The listing builds one solid part. Answer for the finished solid, in the listing's coordinates (mm). Face numbers are marked on the shaded views. A direction names the side the tool comes from. Give positions to 0.01 mm unless a question says otherwise; leave off trailing zeros. Write each loop counter-clockwise with the first axis right and the second up, starting at its lowest first coordinate (ties: lowest second). Pieces come first, ordered by that corner, then holes. Notation, with made-up numbers: (72.5, 50) - (118.5, 50) arc R16 ccw to (118.5, 77) - close; hole circle Ø1 at (71.25, -9). An arc over 180 degrees is marked (long way). Return JSON: item names as keys, results as strings.
from build123d import *

# Parameters (mm, degrees)
SKETCH1_R           = 55.88
BOSS_EXTRUDE1_DEPTH = 23.495
SKETCH2_R           = 66.675
BOSS_EXTRUDE2_DEPTH = 13.97
FILLET1_R           = 7.62
SKETCH3_R           = 2.8575
CUT_EXTRUDE1_DEPTH  = 38.465
CIRPATTERN1_COUNT   = 8
SKETCH4_R           = 38.735
CUT_EXTRUDE2_DEPTH  = 10.795
SKETCH5_R           = 34.4043
CUT_EXTRUDE3_DEPTH  = 40.894


with BuildPart() as part:
    # Sketch1 → Boss-Extrude1 (new body)
    with BuildSketch(Plane(origin=(0, 0, 0), x_dir=(1, 0, 0), z_dir=(0, 1, 0))):
        Circle(SKETCH1_R)
    extrude(amount=BOSS_EXTRUDE1_DEPTH)

    # Sketch2 → Boss-Extrude2 (add)
    with BuildSketch(Plane(origin=(0, 23.495, 0), x_dir=(1, 0, 0), z_dir=(0, 1, 0))):
        Circle(SKETCH2_R)
    extrude(amount=BOSS_EXTRUDE2_DEPTH)

    # Fillet1
    fillet1_edges = [part.edges().sort_by_distance(p)[0] for p in [
        (-55.88, 23.495, 0),
    ]]
    fillet(fillet1_edges, radius=FILLET1_R)

    # Sketch3 → Cut-Extrude1 (cut, through all)
    with BuildSketch(Plane(origin=(0, 37.465, 0), x_dir=(1, 0, 0), z_dir=(0, 1, 0))):
        with Locations((0, 61.2775)):
            Circle(SKETCH3_R)
    cut_extrude1 = extrude(amount=-CUT_EXTRUDE1_DEPTH, mode=Mode.SUBTRACT)

    # CirPattern1: Cut-Extrude1 ×8 about axis
    cirpattern1_axis = Axis((0, 0, 0), (0, 1, 0))
    for i in range(1, CIRPATTERN1_COUNT):
        add(cut_extrude1.rotate(cirpattern1_axis, i * 360 / CIRPATTERN1_COUNT), mode=Mode.SUBTRACT)

    # Sketch4 → Cut-Extrude2 (cut)
    with BuildSketch(Plane(origin=(0, 37.465, 0), x_dir=(1, 0, 0), z_dir=(0, 1, 0))):
        Circle(SKETCH4_R)
    extrude(amount=-CUT_EXTRUDE2_DEPTH, mode=Mode.SUBTRACT)

    # Sketch5 → Cut-Extrude3 (cut)
    with BuildSketch(Plane(origin=(0, 26.67, 0), x_dir=(1, 0, 0), z_dir=(0, 1, 0))):
        Circle(SKETCH5_R)
    extrude(amount=-CUT_EXTRUDE3_DEPTH, mode=Mode.SUBTRACT)


solid = part.part
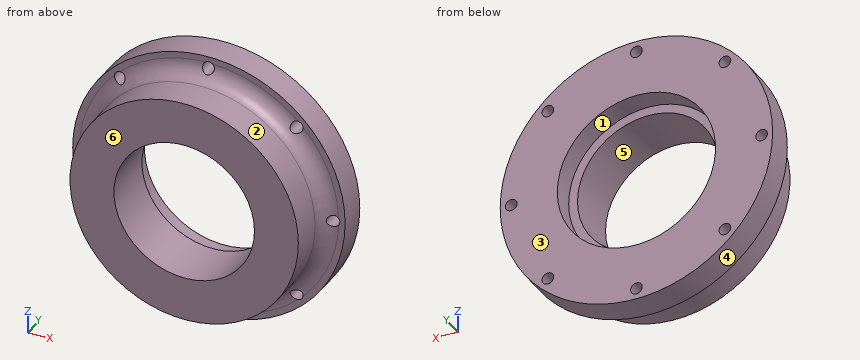
Item 1: Consider L1, parallel to Z at x = 0, y = 30.5 (3 decimals); L2, parallel to X at y = 26, z = 0 (3 decimals). Determine where each line is inside the solid, lowest interval first.
Answer below:
{"L1": "z = -66.675 to -64.135, -58.42 to -38.735, 38.735 to 58.42, 64.135 to 66.675", "L2": "x = -66.675 to -64.135, -58.42 to -34.404, 34.404 to 58.42, 64.135 to 66.675"}
Item 2: The mould has two halves that part along X. Classify the marked faces 4, 5 and 6: +X half, -X half, draft (parallel to the pull), parting line (faces both ways), or undercut.
Answer below:
{"face 4": "parting line", "face 5": "undercut", "face 6": "draft"}
Item 3: A cutting plane is placed at B-B on z = 0. Determine the outline of the cut face in (x, y) (3 decimals), then the cut area to 3 significant figures.
Answer below:
{"outline": "(-66.675, 23.495) - (-64.135, 23.495) - (-64.135, 37.465) - (-66.675, 37.465) - close; (-58.42, 21.555) arc R7.62 cw to (-55.88, 15.875) - (-55.88, 0) - (-34.404, 0) - (-34.404, 26.67) - (-38.735, 26.67) - (-38.735, 37.465) - (-58.42, 37.465) - close; (34.404, 0) - (55.88, 0) - (55.88, 15.875) arc R7.62 cw to (58.42, 21.555) - (58.42, 37.465) - (38.735, 37.465) - (38.735, 26.67) - (34.404, 26.67) - close; (64.135, 23.495) - (66.675, 23.495) - (66.675, 37.465) - (64.135, 37.465) - close", "area": "1,680 mm²"}
Item 4: For the marked faces 1, 2 and 3, determine the directions among +Z, -Z, +X, -X, +Y, -Y from which every point of the face is accessible in a straight line to the end or side of a thin tool.
Answer below:
{"face 1": "+Y", "face 2": "-Y", "face 3": "+Z, -Z, +X, -X, +Y"}
Item 5: Flat-ended cylindrical pins translate along their axes: P1, Ø7.5, axis at x = 61.28, z = 0, coming from the -Y side; P2, Ø9, axis at x = 0, z = 61.28, coming from the -Y side; P3, Ø4, axis at x = -6, y = 19, coming from the +Z side. Find the tip coordinate at first contact, or state that the pin passes through.
Answer below:
{"P1": "stops at y = 20.61", "P2": "stops at y = 19.47", "P3": "stops at z = 57.56"}
Item 6: A cutting plane is placed at D-D on y = 11.5. Determine the outline of the cut face in (x, z), then the cut area to 3 significant figures.
Answer below:
{"outline": "circle Ø111.76 at (0, 0); hole circle Ø68.81 at (0, 0)", "area": "6,090 mm²"}
Item 7: A cutting plane is placed at A-A on x = 0. Determine the outline of the cut face in (y, z) (3 decimals).
Answer below:
{"outline": "(0, -55.88) - (15.875, -55.88) arc R7.62 cw to (21.555, -58.42) - (37.465, -58.42) - (37.465, -38.735) - (26.67, -38.735) - (26.67, -34.404) - (0, -34.404) - close; (0, 34.404) - (26.67, 34.404) - (26.67, 38.735) - (37.465, 38.735) - (37.465, 58.42) - (21.555, 58.42) arc R7.62 cw to (15.875, 55.88) - (0, 55.88) - close; (23.495, -66.675) - (37.465, -66.675) - (37.465, -64.135) - (23.495, -64.135) - close; (23.495, 64.135) - (37.465, 64.135) - (37.465, 66.675) - (23.495, 66.675) - close"}
Item 8: A cutting plane is placed at C-C on y = 33. Give the number of separate pieces and of enclosed holes in the cut face, then the cut area to 3 significant figures.
Answer below:
{"separate pieces": "1", "enclosed holes": "9", "area": "9,050 mm²"}
